Read the model definition and answer for the solid it produces. Units are mm, in the model's axes. Face numbers are marked on the shaded views. A direction names the side the tool comes from. Round coordinates to 2 decimals unless told otherwise and drop trailing zeros. Order: outer loops, then holes, each group sorted by start corner. A loop starts at its lowest first (then second) coordinate and runs counter-clockwise, first axis right, second up. Notation, with made-up numbers: (72, 33.5) - (107, 33.5) arc R31 ccw to (107, 61.5) - close; hole circle Ø5 at (-11, -24). An arc over 180 degrees is marked (long way). Answer as a JSON object with one key per item and string values. Group by question number.
Q1. A cutting plane is placed at A-A on y = 30. Determine the outline of the cut face in (x, z) (3 decimals).
Q2. Consider line 1 (X direction, y = 8.5, z = 3) (3 decimals); line 2 (Y direction, x = -46, z = 0); line 3 (X direction, y = 51, z = -13.5). Determine where each line is inside the solid, lowest interval first.
Q3. A cutting plane is placed at B-B on y = 15.67. Determine the outline of the cut face in (x, z) (3 decimals), and give its area (3 significant figures).
Q4. A cutting plane is placed at C-C on x = 7. Determine the outline of the cut face in (y, z).
Q5. Given pin 1 Ø0.5 at (y, z) = (80, -14.5) entering from -X; pin 2 Ø7.5 at (y, z) = (23, -2) entering from -X (3 decimals); pin 3 Ø9 at (x, y) = (45.5, 22) entering from -Z, each flat-ended and moving along its own axis, determine where each tip first touches the part or whether it passes through.
Q6. A cutting plane is placed at D-D on y = 4. Determine the outline of the cut face in (x, z) (3 decimals), and give its area (3 significant figures).
Q7. A tool of negligible diameter and unlimited length cuts with its end or side. For the marked faces 4, 5, 6 and 7, from which of +Z, -Z, +X, -X, +Y, -Y can it reach the whole face along a straight path? Write none if from no direction.
Q8. The mould has two halves that part along X. Classify the marked faces 1, 2 and 3: pulls with the +X half, pulls with the -X half, needs draft (parallel to the pull), parting line crosses it, or undercut.
```python
from build123d import *

# Parameters (mm, degrees)
BOSS_EXTRU_1_DEPTH                    = 40.5
BOSS_EXTRU_1_DEPTH_BACK               = 5
ESQUISSE1_W                           = 8
ESQUISSE1_H                           = 24.5
BOSS_EXTRU_1_2_DEPTH                  = 40.5
BOSS_EXTRU_1_2_DEPTH_BACK             = 5
ESQUISSE3_R                           = 3.2
ENL_V_MAT_EXTRU_1_DEPTH               = 10.5
ESQUISSE4_W                           = 12.5
ESQUISSE4_H                           = 23
ENL_V_MAT_EXTRU_2_DEPTH               = 10.5
ESQUISSE5_W                           = 8
ESQUISSE5_H                           = 63.6
BOSS_EXTRU_2_DEPTH                    = 15
BOSS_EXTRU_2_2_DEPTH                  = 15
ENL_V_MAT_EXTRU_3_DEPTH               = 156.691080348
ENL_V_START                           = -115.8
ENL_V_MAT_EXTRU_6_DEPTH               = 17.675
ENL_V_START_2                         = -17.675
ENL_V_MAT_EXTRU_6_2_DEPTH             = 17.675
BOSS_EXTRU_3_DEPTH                    = 106.5
ENL_VEMENT_START                      = -22.25
ENL_VEMENT_DE_MATI_RE_BALAYAGE1_DEPTH = 63.6
ENL_VEMENT_DE_MATI_RE_BALAYAGE2_DEPTH = 63.6
ENL_V_MAT_EXTRU_11_DEPTH              = 14
ESQUISSE14_R                          = 1
ENL_V_MAT_EXTRU_12_DEPTH              = 14


with BuildPart() as part:
    # Esquisse1 → Boss.-Extru.1 (new, two sides: drawn at the far end of the back side and taken through both)
    with BuildSketch(Plane(origin=(0, 0, 0), x_dir=(1, 0, 0), z_dir=(0, 1, 0)).offset(-BOSS_EXTRU_1_DEPTH_BACK)):
        with Locations((-44.225, 0)):
            Rectangle(ESQUISSE1_W, ESQUISSE1_H)
    extrude(amount=BOSS_EXTRU_1_DEPTH + BOSS_EXTRU_1_DEPTH_BACK)

    # Esquisse3 → Enlèv. mat.-Extru.1 (cut)
    with BuildSketch(Plane.ZY.offset(48.225)):
        with Locations((0, 15.67)):
            Circle(ESQUISSE3_R)
    extrude(amount=-ENL_V_MAT_EXTRU_1_DEPTH, mode=Mode.SUBTRACT)


with BuildPart() as body_2:
    # Esquisse1 → Boss.-Extru.1 2 (new, two sides: drawn at the far end of the back side and taken through both)
    with BuildSketch(Plane(origin=(0, 0, 0), x_dir=(1, 0, 0), z_dir=(0, 1, 0)).offset(-BOSS_EXTRU_1_2_DEPTH_BACK)):
        with Locations((44.225, 0)):
            Rectangle(ESQUISSE1_W, ESQUISSE1_H)
    extrude(amount=BOSS_EXTRU_1_2_DEPTH + BOSS_EXTRU_1_2_DEPTH_BACK)

    # Esquisse4 → Enlèv. mat.-Extru.2 (cut)
    with BuildSketch(Plane(origin=(48.225, 0, 0), x_dir=(0, 0, -1), z_dir=(1, 0, 0))):
        with Locations((0, 21.5)):
            Rectangle(ESQUISSE4_W, ESQUISSE4_H)
    extrude(amount=-ENL_V_MAT_EXTRU_2_DEPTH, mode=Mode.SUBTRACT)


with BuildPart() as body_3:
    # Esquisse5 → Boss.-Extru.2 (new body)
    with BuildSketch(Plane(origin=(0, 80.5, 0), x_dir=(1, 0, 0), z_dir=(0, 1, 0))):
        with Locations((-53.9, -9.55)):
            Rectangle(ESQUISSE5_W, ESQUISSE5_H)
    extrude(amount=BOSS_EXTRU_2_DEPTH)


with BuildPart() as body_4:
    # Esquisse5 → Boss.-Extru.2 2 (new body)
    with BuildSketch(Plane(origin=(0, 80.5, 0), x_dir=(1, 0, 0), z_dir=(0, 1, 0))):
        with Locations((53.9, -9.55)):
            Rectangle(ESQUISSE5_W, ESQUISSE5_H)
    extrude(amount=BOSS_EXTRU_2_2_DEPTH)


with BuildPart() as enl_v_mat_extru_3_tool:
    # Esquisse6 → Enlèv. mat.-Extru.3 (new, through all)
    with BuildSketch(Plane.ZY.offset(57.9)):
        with BuildLine():
            Line((-19.215648746, 94.3), (-5.284351254, 94.3))
            ThreePointArc((-5.284351254, 94.3), (-4.134351254, 93.15), (-5.284351254, 92))
            Line((-5.284351254, 92), (-19.215648746, 92))
            ThreePointArc((-19.215648746, 92), (-20.365648746, 93.15), (-19.215648746, 94.3))
        make_face()
        with BuildLine():
            Line((23.784351254, 94.3), (37.715648746, 94.3))
            ThreePointArc((37.715648746, 94.3), (38.865648746, 93.15), (37.715648746, 92))
            Line((37.715648746, 92), (23.784351254, 92))
            ThreePointArc((23.784351254, 92), (22.634351254, 93.15), (23.784351254, 94.3))
        make_face()
    extrude(amount=-ENL_V_MAT_EXTRU_3_DEPTH)


with BuildPart() as body_3_1:
    add(body_3.part)

    # Enlèv. mat.-Extru.3: cut by enl_v_mat_extru_3_tool
    add(enl_v_mat_extru_3_tool.part, mode=Mode.SUBTRACT)


    add(part.part)  # lissage2 joins it to this body
    # loft from a face of the part (lissage2)
    loft([body_3_1.faces().sort_by_distance((-53.9, 80.5, 9.55))[0], body_3_1.faces().sort_by_distance((-44.225, 40.5, 0))[0]])

    # Enl_v. mat.-Extru.6 2 outline → Enl_v. mat.-Extru.6 2 (cut)
    with BuildSketch(Plane.ZY.offset(57.9).offset(ENL_V_START_2)):
        Polygon((16.7851704, 58.061718477), (33.416643679, 82.714263273), (13.314021784, 65.095678551), align=None)
        Polygon((-7.878685189, 46.521708187), (8.999873816, 46.521708187), (15.109936371, 55.57854809), (11.118967449, 63.171862295), align=None)
        Polygon((3.513606596, 84.955309113), (12.07666079, 67.60307561), (31.90475538, 84.955309113), align=None)
        Polygon((-1.093401297, 84.955309113), (-15.094337023, 84.955309113), (-9.967028833, 48.311900258), align=None)
        Polygon((9.825440903, 65.632957253), (0.873750807, 82.664659801), (-6.767009008, 51.112345403), align=None)
    extrude(amount=ENL_V_MAT_EXTRU_6_2_DEPTH, mode=Mode.SUBTRACT)



with BuildPart() as body_4_1:
    add(body_4.part)

    # Enlèv. mat.-Extru.3: cut by enl_v_mat_extru_3_tool
    add(enl_v_mat_extru_3_tool.part, mode=Mode.SUBTRACT)


    add(body_2.part)  # lissage1 joins it to this body
    # loft from a face of the part (lissage1)
    loft([body_4_1.faces().sort_by_distance((53.9, 80.5, 9.55))[0], body_4_1.faces().sort_by_distance((44.225, 40.5, 0))[0]])

    # Enlèv. mat.-Extru.6: read off the stored shape, not the designer's step
    # Enlèv. mat.-Extru.6 outline → Enlèv. mat.-Extru.6 (cut)
    with BuildSketch(Plane.ZY.offset(57.9).offset(ENL_V_START)):
        Polygon((16.7851704, 58.061718477), (33.416643679, 82.714263273), (13.314021784, 65.095678551), align=None)
        Polygon((-7.878685189, 46.521708187), (8.999873816, 46.521708187), (15.109936371, 55.57854809), (11.118967449, 63.171862295), align=None)
        Polygon((3.513606596, 84.955309113), (12.07666079, 67.60307561), (31.90475538, 84.955309113), align=None)
        Polygon((-1.093401297, 84.955309113), (-15.094337023, 84.955309113), (-9.967028833, 48.311900258), align=None)
        Polygon((9.825440903, 65.632957253), (0.873750807, 82.664659801), (-6.767009008, 51.112345403), align=None)
    extrude(amount=ENL_V_MAT_EXTRU_6_DEPTH, mode=Mode.SUBTRACT)


with BuildPart() as body_3_2:
    add(body_3_1.part)

    add(body_4_1.part)  # Boss.-Extru.3 merges body 4
    # Esquisse9 → Boss.-Extru.3 (add)
    with BuildSketch(Plane.ZY.offset(-49.9)):
        Polygon((-22.25, 86.627151597), (-15.29778178, 86.627151597), (-8.984735346, 40.434496389), (-12.141258563, 40.434496389), (-22.25, 80.5), align=None)
    extrude(amount=BOSS_EXTRU_3_DEPTH)

    # Enlèvement de matière-Balayage1: read off the stored shape, not the designer's step
    # Enlèvement de matière-Balayage1 outline → Enlèvement de matière-Balayage1 (cut)
    with BuildSketch(Plane.XY.offset(ENL_VEMENT_START)):
        Polygon((49.9, 47.425064599), (48.225, 40.5), (48.225, 40.434496389), (49.9, 40.434496389), align=None)
    extrude(amount=ENL_VEMENT_DE_MATI_RE_BALAYAGE1_DEPTH, mode=Mode.SUBTRACT)

    # Enlèvement de matière-Balayage2: read off the stored shape, not the designer's step
    # Enlèvement de matière-Balayage2 outline → Enlèvement de matière-Balayage2 (cut)
    with BuildSketch(Plane.XY.offset(ENL_VEMENT_START)):
        Polygon((-48.225, 40.5), (-56.6, 75.125322997), (-56.6, 40.434496389), (-48.225, 40.434496389), align=None)
    extrude(amount=ENL_VEMENT_DE_MATI_RE_BALAYAGE2_DEPTH, mode=Mode.SUBTRACT)

    # Esquisse11 → Enlèv. mat.-Extru.11 (cut)
    with BuildSketch(Plane(origin=(0, -0.46401808, -3.395227235), x_dir=(1, 0, 0), z_dir=(0, 0.13540901456567775, 0.9907897853603217))):
        with BuildLine():
            Line((-3.287535233, 83.840431949), (-22.194472995, 83.840431949))
            ThreePointArc((-22.194472995, 83.840431949), (-29.253068949, 82.405282441), (-35.190824132, 78.327722591))
            Line((-35.190824132, 78.327722591), (-21.755006049, 51.469546885))
            Line((-21.755006049, 51.469546885), (-3.287535233, 83.840431949))
        make_face()
        with BuildLine():
            Line((-22.194472995, 47.688497503), (-39.849249541, 69.643827584))
            ThreePointArc((-39.849249541, 69.643827584), (-36.281059291, 54.43712269), (-22.194472995, 47.688497503))
        make_face()
        Polygon((-1.60521279, 82.498170098), (-19.443998314, 47.688497503), (18.984093957, 47.688497503), (-0.418307097, 82.498170098), align=None)
        with BuildLine():
            Line((20.617642495, 83.840431949), (1.70297306, 83.840431949))
            Line((1.70297306, 83.840431949), (21.304692687, 50.51147286))
            Line((21.304692687, 50.51147286), (33.613993633, 78.327722591))
            ThreePointArc((33.613993633, 78.327722591), (27.676238449, 82.405282441), (20.617642495, 83.840431949))
        make_face()
        with BuildLine():
            ThreePointArc((22.784876191, 47.818888972), (35.359080989, 55.303557395), (38.272419041, 69.643827584))
            Line((38.272419041, 69.643827584), (22.784876191, 47.818888972))
        make_face()
    extrude(amount=-ENL_V_MAT_EXTRU_11_DEPTH, mode=Mode.SUBTRACT)

    # Esquisse14 → Enlèv. mat.-Extru.12 (cut)
    with BuildSketch(Plane.ZY.offset(-40.225)):
        with Locations((0, 34.5)):
            Circle(ESQUISSE14_R)
        with Locations(Location((0, 8.5, 0), (0, 0, 180))):
            Circle(ESQUISSE14_R)
    extrude(amount=-ENL_V_MAT_EXTRU_12_DEPTH, mode=Mode.SUBTRACT)


solid = body_3_2.part
```
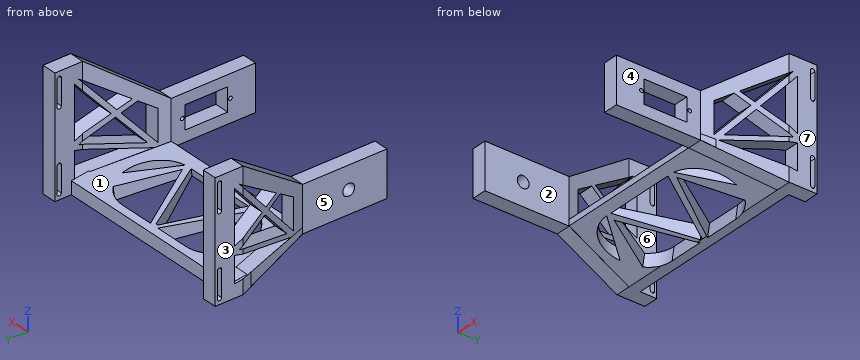
Result set:
{
 "1": {"outline": "(-48.225, -12.25) - (-40.225, -12.25) - (-40.225, 12.25) - (-48.225, 12.25) - close; (40.225, -12.25) - (48.225, -12.25) - (48.225, -6.25) - (40.225, -6.25) - close; (40.225, 6.25) - (48.225, 6.25) - (48.225, 12.25) - (40.225, 12.25) - close"},
 "2": {"line 1": "x = -48.225 to -40.225, 40.225 to 48.225", "line 2": "y = -5 to 12.47, 18.87 to 46.52, 53.43 to 57.03", "line 3": "x = -50.76 to -34.32, -25.95 to -22.2, -21.25 to -17.05, 16.38 to 20.22, 22.12 to 26.01, 32.74 to 50.76"},
 "3": {"outline": "(-48.225, -12.25) - (-40.225, -12.25) - (-40.225, -3.2) - (-48.225, -3.2) - close; (-48.225, 3.2) - (-40.225, 3.2) - (-40.225, 12.25) - (-48.225, 12.25) - close; (40.225, -12.25) - (48.225, -12.25) - (48.225, -6.25) - (40.225, -6.25) - close; (40.225, 6.25) - (48.225, 6.25) - (48.225, 12.25) - (40.225, 12.25) - close", "area": "241 mm²"},
 "4": {"outline": "(40.43, -12.14) - (46.27, -13.61) - (46.79, -9.85) - (40.43, -8.98) - close; (67.25, -18.91) - (72.76, -20.3) - (73.68, -13.53) - (68.09, -12.76) - close; (81.58, -22.25) - (86.63, -22.25) - (86.63, -15.3) - (82.6, -14.75) - close"},
 "5": {"pin 1": "stops at x = -57.84", "pin 2": "stops at x = -48.225", "pin 3": "stops at z = -12.25"},
 "6": {"outline": "(-48.225, -12.25) - (-40.225, -12.25) - (-40.225, 12.25) - (-48.225, 12.25) - close; (40.225, -12.25) - (48.225, -12.25) - (48.225, 12.25) - (40.225, 12.25) - close", "area": "392 mm²"},
 "7": {"face 4": "+Z, -Z, +X, -Y", "face 5": "+Z, -Z, -X, -Y", "face 6": "+Z, +Y", "face 7": "+Z, -Z, +X, +Y, -Y"},
 "8": {"face 1": "undercut", "face 2": "undercut", "face 3": "pulls with the -X half"}
}
